For this review, take the finished solid that the model builds, in its own axes (mm). Coordinates: 2 decimals unless noted, no trailing zeros. Write each loop counter-clockwise with the first axis right and the second up, starting at its lowest first coordinate (ties: lowest second). Pieces come first, ordered by that corner, then holes. Notation, with made-up numbers: (-25.75, 4) - (1.25, 4) arc R14 cw to (1.25, 25) - close; hole circle Ø4 at (-39.5, 18). An arc over 180 degrees is marked (long way). Use one line per item in the form item = value. Start each with the question number.
1) We need section B-B (z = 0.55). Count the separate pieces of the cut face and the enclosed holes in it, plus the area to 3 significant figures.
2) We need section C-C (x = 58.5). Give the boundary of the cut face in (y, z).
3) For L1, parallel to Y at x = 58.5, z = 0.85; L2, parallel to X at y = 81.5, z = 1.4; L3, parallel to X at y = 112.5, z = 0.75, list the stretches that pass through material, from the lowest coordinate up. Write a range as from..to.
4) We need section A-A (y = 170). Give the boundary of the cut face in (x, z).
5) Insertion check: P1, Ø0.6, axis at y = 148, z = 1.5, coming from the +X side; P2, Ø0.6, axis at x = 30.5, z = 1.5, coming from the +Y side; P3, Ø1, axis at y = 25.5, z = 0.5, coming from the +X side. Each pin has a flat end and moves straight along its axis. Give the tip position at first contact, or say it passes through.
6) We need section D-D (y = 75). Give the boundary of the cut face in (x, z), plus the area to 3 significant figures.
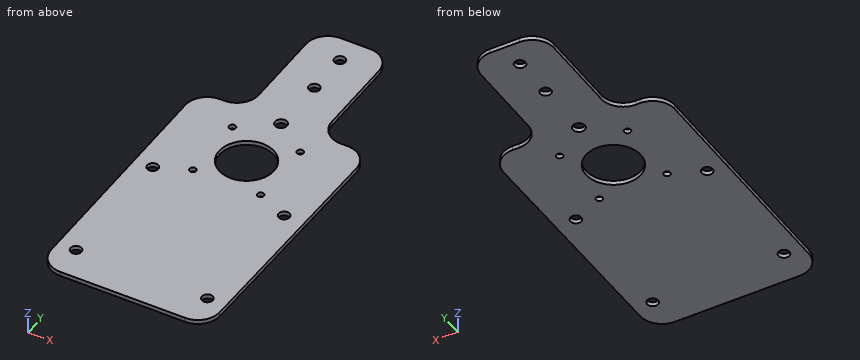
```python
from build123d import *

# Parameters (mm, degrees)
SKETCH1_W           = 117
SKETCH1_H           = 200
BOSS_EXTRUDE1_DEPTH = 2
CUT_EXTRUDE1_DEPTH  = 2
SKETCH3_R           = 2.5
SKETCH3_R_2         = 1.5
SKETCH3_R_3         = 12.5
SKETCH3_R_4         = 2.75
CUT_EXTRUDE2_DEPTH  = 30
FILLET1_R           = 20
CUT_EXTRUDE3_DEPTH  = 10
FILLET2_R           = 10
CUT_EXTRUDE4_DEPTH  = 10
FILLET3_R           = 10
CUT_EXTRUDE5_DEPTH  = 10
FILLET4_R           = 10


with BuildPart() as part:
    # Sketch1 → Boss-Extrude1 (new body)
    with BuildSketch(Plane.XY):
        with Locations((58.5, 100)):
            Rectangle(SKETCH1_W, SKETCH1_H)
    extrude(amount=BOSS_EXTRUDE1_DEPTH)

    # Sketch2 → Cut-Extrude1 (cut)
    with BuildSketch(Plane.XY.offset(2)):
        Polygon((0, 120), (40, 200), (0, 200), align=None)
        Polygon((77, 200), (117, 120), (117, 200), align=None)
    extrude(amount=-CUT_EXTRUDE1_DEPTH, mode=Mode.SUBTRACT)

    # Sketch3 → Cut-Extrude2 (cut)
    with BuildSketch(Plane.XY.offset(2)):
        with Locations((58.5, 170)):
            Circle(SKETCH3_R)
        with Locations((58.5, 150)):
            Circle(SKETCH3_R)
        with Locations((28.5, 15)):
            Circle(SKETCH3_R)
        with Locations((88.5, 15)):
            Circle(SKETCH3_R)
        with Locations((28.5, 75)):
            Circle(SKETCH3_R)
        with Locations((88.5, 75)):
            Circle(SKETCH3_R)
        with Locations((43, 112.5)):
            Circle(SKETCH3_R_2)
        with Locations((43, 81.5)):
            Circle(SKETCH3_R_2)
        with Locations((74, 81.5)):
            Circle(SKETCH3_R_2)
        with Locations((74, 112.5)):
            Circle(SKETCH3_R_2)
        with Locations((58.5, 97)):
            Circle(SKETCH3_R_3)
        with Locations((58.5, 124)):
            Circle(SKETCH3_R_4)
    extrude(amount=-CUT_EXTRUDE2_DEPTH, mode=Mode.SUBTRACT)

    # Fillet1
    fillet1_edges = [part.edges().sort_by_distance(p)[0] for p in [
        (0, 120, 1),
        (40, 200, 1),
        (117, 120, 1),
        (77, 200, 1),
        (117, 0, 1),
        (0, 0, 1),
    ]]
    fillet(fillet1_edges, radius=FILLET1_R)

    # Sketch4 → Cut-Extrude3 (cut)
    with BuildSketch(Plane(origin=(0, 0, 0), x_dir=(-1, 0, 0), z_dir=(0, 0, -1))):
        with BuildLine():
            Line((-97, 0), (-98.708203932, 156.583592135))
            Line((-98.708203932, 156.583592135), (-114.88854382, 124.22291236))
            ThreePointArc((-114.88854382, 124.22291236), (-116.464979789, 119.873698861), (-117, 115.27864045))
            Line((-117, 115.27864045), (-117, 20))
            ThreePointArc((-117, 20), (-111.142135624, 5.857864376), (-97, 0))
        make_face()
        with BuildLine():
            Line((-20, 0), (-20, 160))
            Line((-20, 160), (-18.291796068, 156.583592135))
            Line((-18.291796068, 156.583592135), (-2.11145618, 124.22291236))
            ThreePointArc((-2.11145618, 124.22291236), (-0.535020211, 119.873698861), (0, 115.27864045))
            Line((0, 115.27864045), (0, 20))
            ThreePointArc((0, 20), (-5.857864376, 5.857864376), (-20, 0))
        make_face()
    extrude(amount=-CUT_EXTRUDE3_DEPTH, mode=Mode.SUBTRACT)

    # Fillet2
    fillet2_edges = [part.edges().sort_by_distance(p)[0] for p in [
        (97, 0, 1),
        (20, 0, 1),
        (98.708203932, 156.583592135, 1),
        (20, 160, 1),
    ]]
    fillet(fillet2_edges, radius=FILLET2_R)

    # Sketch5 → Cut-Extrude4 (cut)
    with BuildSketch(Plane(origin=(0, 0, 0), x_dir=(-1, 0, 0), z_dir=(0, 0, -1))):
        with BuildLine():
            Line((-75.153942467, 125.055763262), (-75.153942467, 197.013016167))
            ThreePointArc((-75.153942467, 197.013016167), (-79.402826552, 193.49217851), (-82.527864045, 188.94427191))
            Line((-82.527864045, 188.94427191), (-97.626690246, 158.746619509))
            ThreePointArc((-97.626690246, 158.746619509), (-98.427295018, 156.518894044), (-98.681823334, 154.165397904))
            Line((-98.681823334, 154.165397904), (-98.364260097, 125.055763262))
            Line((-98.364260097, 125.055763262), (-75.153942467, 125.055763262))
        make_face()
        with BuildLine():
            ThreePointArc((-34.472135955, 188.94427191), (-37.597173448, 193.49217851), (-41.846057533, 197.013016167))
            Line((-41.846057533, 197.013016167), (-41.846057533, 125.055763262))
            Line((-41.846057533, 125.055763262), (-20, 125.055763262))
            Line((-20, 125.055763262), (-20, 157.639320225))
            ThreePointArc((-20, 157.639320225), (-20.267510105, 159.93684943), (-21.05572809, 162.11145618))
            Line((-21.05572809, 162.11145618), (-34.472135955, 188.94427191))
        make_face()
    extrude(amount=-CUT_EXTRUDE4_DEPTH, mode=Mode.SUBTRACT)

    # Fillet3
    fillet3_edges = [part.edges().sort_by_distance(p)[0] for p in [
        (75.153942467, 197.013016167, 1),
        (41.846057533, 197.013016167, 1),
        (75.153942467, 125.055763262, 1),
        (98.364260097, 125.055763262, 1),
        (41.846057533, 125.055763262, 1),
        (20, 125.055763262, 1),
    ]]
    fillet(fillet3_edges, radius=FILLET3_R)

    # Sketch6 → Cut-Extrude5 (cut)
    with BuildSketch(Plane(origin=(0, 0, 0), x_dir=(-1, 0, 0), z_dir=(0, 0, -1))):
        with BuildLine():
            Line((-75.153942467, 189.986749418), (-75.153942467, 182))
            Line((-75.153942467, 182), (-41.846057533, 182))
            Line((-41.846057533, 182), (-41.846057533, 189.986749418))
            ThreePointArc((-41.846057533, 189.986749418), (-44.595325762, 196.873467707), (-51.33143529, 199.973498837))
            ThreePointArc((-51.33143529, 199.973498837), (-51.845886972, 199.993373612), (-52.360679775, 200))
            Line((-52.360679775, 200), (-64.639320225, 200))
            ThreePointArc((-64.639320225, 200), (-65.154113028, 199.993373612), (-65.66856471, 199.973498837))
            ThreePointArc((-65.66856471, 199.973498837), (-72.404674238, 196.873467707), (-75.153942467, 189.986749418))
        make_face()
    extrude(amount=-CUT_EXTRUDE5_DEPTH, mode=Mode.SUBTRACT)

    # Fillet4
    fillet4_edges = [part.edges().sort_by_distance(p)[0] for p in [
        (41.846057533, 182, 1),
        (75.153942467, 182, 1),
    ]]
    fillet(fillet4_edges, radius=FILLET4_R)


solid = part.part
```
Determined:
q1.separate_pieces = 1
q1.enclosed_holes = 12
q1.area = 10,900 mm²
q2.outline = (0, 0) - (84.5, 0) - (84.5, 2) - (0, 2) - close; (109.5, 0) - (121.25, 0) - (121.25, 2) - (109.5, 2) - close; (126.75, 0) - (147.5, 0) - (147.5, 2) - (126.75, 2) - close; (152.5, 0) - (167.5, 0) - (167.5, 2) - (152.5, 2) - close; (172.5, 0) - (182, 0) - (182, 2) - (172.5, 2) - close
q3.L1 = 0..84.5, 109.5..121.25, 126.75..147.5, 152.5..167.5, 172.5..182
q3.L2 = 20..41.5, 44.5..72.5, 75.5..97.89
q3.L3 = 20..41.5, 44.5..72.5, 75.5..98.23
q4.outline = (41.85, 0) - (56, 0) - (56, 2) - (41.85, 2) - close; (61, 0) - (75.15, 0) - (75.15, 2) - (61, 2) - close
q5.P1 = 75.15
q5.P2 = 125.06
q5.P3 = 97.28
q6.outline = (20, 0) - (26, 0) - (26, 2) - (20, 2) - close; (31, 0) - (86, 0) - (86, 2) - (31, 2) - close; (91, 0) - (97.82, 0) - (97.82, 2) - (91, 2) - close
q6.area = 136 mm²
